from build123d import *

# Parameters (mm, degrees)
SKETCH1_R           = 2.6
SKETCH1_R_2         = 2.15
SKETCH1_R_3         = 5
SKETCH1_R_4         = 2.1
BOSS_EXTRUDE1_DEPTH = 6
FILLET1_R           = 5
FILLET2_R           = 6
FILLET3_R           = 10
FILLET4_R           = 20
FILLET5_R           = 10


with BuildPart() as part:
    # Sketch1 → Boss-Extrude1 (new body)
    with BuildSketch(Plane(origin=(0, 0, 0), x_dir=(1, 0, 0), z_dir=(0, 1, 0))):
        Polygon((159.965380006, 15), (134.965380006, 28), (18, 28), (8, 33), (-2, 33), (-18, 16), (-18, 0), (0, 0), (129.965380006, 0), (159.965380006, 3), align=None)
        with Locations(Location((-11, 10, 0), (0, 0, 270))):
            Circle(SKETCH1_R, mode=Mode.SUBTRACT)
        with Locations(Location((129, 13, 0), (0, 0, 270))):
            Circle(SKETCH1_R_2, mode=Mode.SUBTRACT)
        with Locations(Location((25, 13, 0), (0, 0, 270))):
            Circle(SKETCH1_R_3, mode=Mode.SUBTRACT)
        with Locations(Location((154.965380006, 10, 0), (0, 0, 270))):
            Circle(SKETCH1_R, mode=Mode.SUBTRACT)
        with Locations(Location((1, 26, 0), (0, 0, 270))):
            Circle(SKETCH1_R, mode=Mode.SUBTRACT)
        with Locations(Location((50, 13, 0), (0, 0, 270))):
            Circle(SKETCH1_R_4, mode=Mode.SUBTRACT)
        with Locations(Location((70, 13, 0), (0, 0, 270))):
            Circle(SKETCH1_R_4, mode=Mode.SUBTRACT)
    extrude(amount=BOSS_EXTRUDE1_DEPTH)

    # Fillet1
    fillet1_edges = [part.edges().sort_by_distance(p)[0] for p in [
        (-18, 3, 0),
    ]]
    fillet(fillet1_edges, radius=FILLET1_R)

    # Fillet2
    # the kernel refuses this fillet: 6 mm, written as the material it takes off along each edge
    with BuildSketch(Plane(origin=(159.965380006, -9.106803364, -15), x_dir=(0, 0, 1), z_dir=(0, 1, 0))) as fillet2_piece_1:
        with BuildLine():
            CenterArc((FILLET2_R * 0.607120224288, -FILLET2_R), FILLET2_R, 90, 62.525568374)
            Line((-FILLET2_R * 0.280096576946, -FILLET2_R * 0.538647263358), (0, 0))
            Line((0, 0), (FILLET2_R * 0.607120224288, 0))
        make_face()
    extrude(amount=24.213606729, mode=Mode.SUBTRACT)
    with BuildSketch(Plane(origin=(159.965380006, -13.574813432, -3), x_dir=(-0.9950371902099892, 0, 0.0995037190209987), z_dir=(0, 1, 0))) as fillet2_piece_2:
        with BuildLine():
            CenterArc((FILLET2_R * 0.904987562112, -FILLET2_R), FILLET2_R, 90, 84.289406863)
            Line((-FILLET2_R * 0.0900496280979, -FILLET2_R * 0.900496280979), (0, 0))
            Line((0, 0), (FILLET2_R * 0.904987562112, 0))
        make_face()
    extrude(amount=33.149626863, mode=Mode.SUBTRACT)
    with BuildSketch(Plane(origin=(129.965380006, -0.748134317, 0), x_dir=(-1, 0, 0), z_dir=(0, 1, 0))) as fillet2_piece_3:
        with BuildLine():
            CenterArc((FILLET2_R * 0.0498756211209, -FILLET2_R), FILLET2_R, 90, 5.710593137)
            Line((-FILLET2_R * 0.0496280979001, -FILLET2_R * 0.00496280979001), (0, 0))
            Line((0, 0), (FILLET2_R * 0.0498756211209, 0))
        make_face()
    extrude(amount=7.496268634, mode=Mode.SUBTRACT)

    # Fillet3
    fillet3_edges = [part.edges().sort_by_distance(p)[0] for p in [
        (-18, 3, -16),
        (-2, 3, -33),
    ]]
    fillet(fillet3_edges, radius=FILLET3_R)

    # Fillet4
    fillet4_edges = [part.edges().sort_by_distance(p)[0] for p in [
        (134.965380006, 3, -28),
    ]]
    fillet(fillet4_edges, radius=FILLET4_R)

    # Fillet5
    fillet5_edges = [part.edges().sort_by_distance(p)[0] for p in [
        (8, 3, -33),
        (18, 3, -28),
    ]]
    fillet(fillet5_edges, radius=FILLET5_R)


solid = part.part
Geometry check sheet. Reference: the model listing, model coordinates, mm. A direction names the side the tool comes from. Round coordinates to 2 decimals unless told otherwise and drop trailing zeros. Loops run counter-clockwise (first coordinate to the right, second up) from the corner with the lowest first, then second, coordinate; pieces in that order, holes last. Notation, with made-up numbers: (9, 37.25) - (46, 37.25) arc R22 ccw to (46, 68.25) - close; hole circle Ø6 at (47.5, 47.25). An arc over 180 degrees is marked (long way). One line per question, with ' | ' between items. Start each with the question number.
1. Cross-section at B-B on y = 0.9. Record the cut outline in (x, z), then the cut area to 3 significant figures.
2. Depth check by flat-ended pin: pin 1 (3 mm diameter, centred on x = 99, y = 4, fed in from -Z); pin 2 (1 mm diameter, centred on y = 5, z = -29, fed in from -X). Enter the tip coordinate at first touch or a pass-through.
3. Draft check along Z on faces 1 (the face through (-1.54, 2.96, -26.56)), 2 (the face through (158.372, 2.958, -4.358)), 3 (the face through (-1.698, 3.042, -32.157)). Enter one of: released by +Z, released by -Z, zero draft, split by the parting line, or undercut.
4. Scan lines: line 1 (X direction, y = 2.65, z = -13); line 2 (Z direction, x = 129, y = 1.35); line 3 (X direction, y = 4, z = -10). Record each from-to range of solid material in increasing order. Write a range as [from, to].
5. Cross-section at C-C on x = 25. Record the cut outline in (y, z).
6. Cross-section at A-A on x = 70. Record the cut outline in (y, z), then the cut area to 3 significant figures.
7. Tool access check on faces 4 (the face through (-10.049, 2.958, -24.448)), 5 (the face through (76, 3, -28)). Record the directions out of +Z, -Z, +X, -X, +Y, -Y that give a thin tool (end or side, any length) a straight path to the whole face; none if there is none.
Taken from the geometry:
1) outline: (-18, -12.03) arc R10 ccw to (-15.28, -18.89) - (-4.96, -29.85) arc R10 ccw to (2.32, -33) - (5.64, -33) arc R10 ccw to (10.11, -31.94) - (15.89, -29.06) arc R10 cw to (20.36, -28) - (130.08, -28) arc R20 ccw to (139.3, -25.74) - (156.73, -16.68) arc R6 ccw to (159.97, -11.36) - (159.97, -8.43) arc R6 ccw to (154.56, -2.46) - (130.26, -0.03) arc R6 ccw to (129.67, 0) - (-13, 0) arc R5 ccw to (-18, -5) - close; hole circle Ø5.2 at (-11, -10); hole circle Ø5.2 at (1, -26); hole circle Ø10 at (25, -13); hole circle Ø4.2 at (50, -13); hole circle Ø4.2 at (70, -13); hole circle Ø4.3 at (129, -13); hole circle Ø5.2 at (154.97, -10) | area: 4,590 mm²
2) pin 1: z = -28 | pin 2: x = -6.24
3) face 1: undercut | face 2: released by +Z | face 3: released by -Z
4) line 1: [-17.95, 20], [30, 47.9], [52.1, 67.9], [72.1, 126.85], [131.15, 159.74] | line 2: [-28, -15.15], [-10.85, 0] | line 3: [-18, -13.6], [-8.4, 21], [29, 152.37], [157.57, 159.97]
5) outline: (0, -28) - (6, -28) - (6, -18) - (0, -18) - close; (0, -8) - (6, -8) - (6, 0) - (0, 0) - close
6) outline: (0, -28) - (6, -28) - (6, -15.1) - (0, -15.1) - close; (0, -10.9) - (6, -10.9) - (6, 0) - (0, 0) - close | area: 143 mm²
7) face 4: -Z, -X, +Y, -Y | face 5: -Z, +X, +Y, -Y
